Input: part model. Units: mm. Frame: model coordinates. A direction names the side the tool comes from. Coordinates: 2 decimals unless noted, no trailing zeros. Order: outer loops, then holes, each group sorted by start corner. A loop starts at its lowest first (then second) coordinate and runs counter-clockwise, first axis right, second up.
from build123d import *

# Parameters (mm, degrees)
EXTRUDE1_DEPTH     = 12.7
SKETCH2_W          = 152.4
SKETCH2_H          = 12.7
EXTRUDE2_DEPTH     = 25.4
MIRROR1_START      = 38.1
MIRROR1_OUTLINE_W  = 152.4
MIRROR1_OUTLINE_H  = 12.7
MIRROR1_DEPTH      = 38.1
MIRROR1_START_2    = 63.5
MIRROR1_2_DEPTH    = 12.7
SKETCH4_R          = 6.35
CUT_EXTRUDE1_DEPTH = 115.3


# Read off the part's stored shape, not the designer's step: Mirror1
with BuildPart() as part:
    # Sketch1 → Extrude1 (new body)
    with BuildSketch(Plane.XY):
        with BuildLine():
            Line((-31.75, 38.1), (31.75, 38.1))
            ThreePointArc((31.75, 38.1), (47.934687961, 12.002969288), (76.2, 0))
            Line((76.2, 0), (76.2, -12.7))
            Line((76.2, -12.7), (-76.2, -12.7))
            Line((-76.2, -12.7), (-76.2, 0))
            ThreePointArc((-76.2, 0), (-47.934687961, 12.002969288), (-31.75, 38.1))
        make_face()
    extrude(amount=EXTRUDE1_DEPTH)

    # Sketch2 → Extrude2 (add)
    with BuildSketch(Plane.XY.offset(12.7)):
        with Locations((0, -6.35)):
            Rectangle(SKETCH2_W, SKETCH2_H)
    extrude(amount=EXTRUDE2_DEPTH)

    # Mirror1 outline → Mirror1 (add)
    with BuildSketch(Plane.XY.offset(MIRROR1_START)):
        with Locations((0, -6.35)):
            Rectangle(MIRROR1_OUTLINE_W, MIRROR1_OUTLINE_H)
    extrude(amount=MIRROR1_DEPTH)

    # Mirror1 2 outline → Mirror1 2 (add)
    with BuildSketch(Plane.XY.offset(MIRROR1_START_2)):
        with BuildLine():
            ThreePointArc((-31.75, 38.1), (-47.934687961, 12.002969288), (-76.2, 0))
            Line((-76.2, 0), (76.2, 0))
            ThreePointArc((76.2, 0), (47.934687961, 12.002969288), (31.75, 38.1))
            Line((31.75, 38.1), (-31.75, 38.1))
        make_face()
    extrude(amount=MIRROR1_2_DEPTH)

    # Sketch4 → Cut-Extrude1 (cut, through all)
    with BuildSketch(Plane(origin=(0, 0, 0), x_dir=(-1, 0, 0), z_dir=(0, 0, -1))):
        with Locations((-19.05, 19.05)):
            Circle(SKETCH4_R)
        with Locations((19.05, 19.05)):
            Circle(SKETCH4_R)
    extrude(amount=-CUT_EXTRUDE1_DEPTH, mode=Mode.SUBTRACT)


solid = part.part
Item 1: Cut plane B-B on z = 72.5. Return loops of the section in (x, y), then the cut area to 3 significant figures.
Response values:
outline: (-76.2, -12.7) - (76.2, -12.7) - (76.2, 0) arc R50.8 cw to (31.75, 38.1) - (-31.75, 38.1) arc R50.8 cw to (-76.2, 0) - close; hole circle Ø12.7 at (-19.05, 19.05); hole circle Ø12.7 at (19.05, 19.05)
area: 5,060 mm2
Item 2: Draft query along X for faces 1 (the face through (19.877, 25.346, 6.261)), 2 (the face through (-1, 0, 38)), 3 (the face through (-22.464, 24.404, 69.761)), 4 (the face through (47.6, 12.29, 6.26)). Return one class per face: pulls with the +X half, pulls with the -X half, needs draft (parallel to the pull), parting line crosses it, or undercut.
Response values:
face 1: undercut
face 2: needs draft
face 3: undercut
face 4: pulls with the +X half
Item 3: Cut plane C-C on y = 17. Return loops of the section in (x, z).
Response values:
outline: (-42.87, 0) - (-25.06, 0) - (-25.06, 12.7) - (-42.87, 12.7) - close; (-42.87, 63.5) - (-25.06, 63.5) - (-25.06, 76.2) - (-42.87, 76.2) - close; (-13.04, 0) - (13.04, 0) - (13.04, 12.7) - (-13.04, 12.7) - close; (-13.04, 63.5) - (13.04, 63.5) - (13.04, 76.2) - (-13.04, 76.2) - close; (25.06, 0) - (42.87, 0) - (42.87, 12.7) - (25.06, 12.7) - close; (25.06, 63.5) - (42.87, 63.5) - (42.87, 76.2) - (25.06, 76.2) - close
Item 4: Ray query, probe 1 along Y at (x, z) = (-19.05, 3); probe 2 along Z at (x, y) = (7, 7.5); probe 3 along X at (y, z) = (19, 71). Return the intervals inside material, ascending.
Response values:
probe 1: y = -12.7 to 12.7, 25.4 to 38.1
probe 2: z = 0 to 12.7, 63.5 to 76.2
probe 3: x = -41.2 to -25.4, -12.7 to 12.7, 25.4 to 41.2
Item 5: Pin query (flat end, axial travel): pin 1 Ø4 at (x, y) = (47.5, 9.5) entering from -Z; pin 2 Ø15 at (x, z) = (-29.5, 36.5) entering from +Y. Return the tip coordinate at first contact, or that it passes through.
Response values:
pin 1: stops at z = 0
pin 2: stops at y = 0
Item 6: Cut plane D-D on y = 32.5. Return loops of the section in (x, z), then the cut area to 3 significant figures.
Response values:
outline: (-33.52, 0) - (33.52, 0) - (33.52, 12.7) - (-33.52, 12.7) - close; (-33.52, 63.5) - (33.52, 63.5) - (33.52, 76.2) - (-33.52, 76.2) - close
area: 1,700 mm2
Item 7: Access query for faces 5 (the face through (19.877, 25.346, 69.761)), 6 (the face through (-1, 15, 63.5)). Directions: +Z, -Z, +X, -X, +Y, -Y. A direction counts if a zero-diameter tool reaches every point of the face in a straight line with its end or side. Return the directions, or none.
Response values:
face 5: +Z, -Z
face 6: +X, -X, +Y
Item 8: Cut plane A-A on x = 19.05. Return loops of the section in (y, z).
Response values:
outline: (-12.7, 0) - (12.7, 0) - (12.7, 12.7) - (0, 12.7) - (0, 63.5) - (12.7, 63.5) - (12.7, 76.2) - (-12.7, 76.2) - close; (25.4, 0) - (38.1, 0) - (38.1, 12.7) - (25.4, 12.7) - close; (25.4, 63.5) - (38.1, 63.5) - (38.1, 76.2) - (25.4, 76.2) - close
